The listing builds one solid part. Answer for the finished solid, in the listing's coordinates (mm). A direction names the side the tool comes from. Give positions to 0.01 mm unless a question says otherwise; leave off trailing zeros. Order: outer loops, then holes, each group sorted by start corner. A loop starts at its lowest first (then second) coordinate and runs counter-clockwise, first axis right, second up. Notation, with made-up numbers: (-36, 83.25) - (-29, 83.25) arc R17 ccw to (-29, 111.25) - close; hole circle Ø8 at (38.5, 79.25). An arc over 180 degrees is marked (long way). Write each question's results on one line, items separated by ' | '. Start each with the question number.
1. Section C-C (z = -12) is taken. Give the vertices of the cut face in (x, y), and give its area (3 significant figures).
2. Find the intervals of material crossed by L1, parallel to X at y = 43, z = 0; L2, parallel to X at y = 44.5, z = 44; L3, parallel to Z at x = -42, y = 34.5, in increasing order.
3. Flat-ended cylindrical pins translate along their axes: pin 1 (2 mm diameter, centred on x = -5.5, z = 67, fed in from +Y); pin 2 (1.5 mm diameter, centred on y = 32.5, z = 55, fed in from +X); pin 3 (3.5 mm diameter, centred on y = 47.5, z = 67.5, fed in from +X). Find the tip coordinate at first contact, or state that the pin passes through.
4. Section D-D (z = 61) is taken. Give the vertices of the cut face in (x, y).
5. Section A-A (y = 7.5) is taken. Give the vertices of the cut face in (x, z).
6. Which of the six approach directions +Z, -Z, +X, -X, +Y, -Y give full straight-line access (tool end or side, diameter ignored) to faces 4 (the face through (-1, 28, -65)), 5 (the face through (-15, 46, 69)), 6 (the face through (66.297, 2.535, -65.986))?
7. Section B-B (x = 34.5) is taken. Give the vertices of the cut face in (y, z), and give its area (3 significant figures).
8. Determine the mould class of faces 1 (the face through (-1, 0, -1)), 2 (the face through (-1, 25, 72)), 3 (the face through (52, 28, 1)) for opening direction Z: released by +Z, released by -Z, zero draft, split by the parting line, or undercut.
from build123d import *

# Parameters (mm, degrees)
SKETCH1_W           = 144
SKETCH1_H           = 144
BOSS_EXTRUDE1_DEPTH = 5
FILLET1_R           = 20
BOSS_EXTRUDE2_START = 45
SKETCH2_W           = 104
SKETCH2_H           = 130
BOSS_EXTRUDE2_DEPTH = 45
SKETCH3_R           = 1.5
CUT_EXTRUDE1_DEPTH  = 13
SKETCH5_W           = 15
SKETCH5_H           = 8
CUT_EXTRUDE2_DEPTH  = 8


with BuildPart() as part:
    # Sketch1 → Boss-Extrude1 (new body)
    with BuildSketch(Plane(origin=(0, 0, 0), x_dir=(1, 0, 0), z_dir=(0, 1, 0))):
        Rectangle(SKETCH1_W, SKETCH1_H)
    extrude(amount=BOSS_EXTRUDE1_DEPTH)

    # Fillet1
    fillet1_edges = [part.edges().sort_by_distance(p)[0] for p in [
        (72, 2.5, 72),
        (-72, 2.5, 72),
        (-72, 2.5, -72),
        (72, 2.5, -72),
    ]]
    fillet(fillet1_edges, radius=FILLET1_R)

    # Sketch2 → Boss-Extrude2 (add)
    with BuildSketch(Plane(origin=(0, 5, 0), x_dir=(1, 0, 0), z_dir=(0, 1, 0)).offset(BOSS_EXTRUDE2_START)):
        with BuildLine():
            Line((-72, 52), (-72, -52))
            ThreePointArc((-72, -52), (-66.142135624, -66.142135624), (-52, -72))
            Line((-52, -72), (52, -72))
            ThreePointArc((52, -72), (66.142135624, -66.142135624), (72, -52))
            Line((72, -52), (72, 62))
            ThreePointArc((72, 62), (69.071067812, 69.071067812), (62, 72))
            Line((62, 72), (-52, 72))
            ThreePointArc((-52, 72), (-66.142135624, 66.142135624), (-72, 52))
        make_face()
        Rectangle(SKETCH2_W, SKETCH2_H, mode=Mode.SUBTRACT)
    extrude(amount=-BOSS_EXTRUDE2_DEPTH)

    # Sketch3 → Cut-Extrude1 (cut)
    with BuildSketch(Plane(origin=(0, 50, 0), x_dir=(1, 0, 0), z_dir=(0, 1, 0))):
        with Locations(Location((-67, 0, 0), (0, 0, 270))):
            Circle(SKETCH3_R)
        with Locations(Location((67, 0, 0), (0, 0, 270))):
            Circle(SKETCH3_R)
    extrude(amount=-CUT_EXTRUDE1_DEPTH, mode=Mode.SUBTRACT)

    # Sketch5 → Cut-Extrude2 (cut)
    with BuildSketch(Plane.XY.offset(72)):
        with Locations((-7.5, 46)):
            Rectangle(SKETCH5_W, SKETCH5_H)
    extrude(amount=-CUT_EXTRUDE2_DEPTH, mode=Mode.SUBTRACT)


solid = part.part
Reported:
1) outline: (-72, 0) - (72, 0) - (72, 50) - (52, 50) - (52, 5) - (-52, 5) - (-52, 50) - (-72, 50) - close | area: 2,520 mm²
2) L1: -72 to -68.5, -65.5 to -52, 52 to 65.5, 68.5 to 72 | L2: -72 to -52, 52 to 72 | L3: -72 to -65, 65 to 72
3) pin 1: y = 42 | pin 2: x = 71.87 | pin 3: x = 66.52
4) outline: (-69.86, 0) - (69.86, 0) - (69.86, 50) - (52, 50) - (52, 5) - (-52, 5) - (-52, 50) - (-69.86, 50) - close
5) outline: (-72, -52) arc R20 ccw to (-52, -72) - (62, -72) arc R10 ccw to (72, -62) - (72, 52) arc R20 ccw to (52, 72) - (-52, 72) arc R20 ccw to (-72, 52) - close; hole (-52, -65) - (52, -65) - (52, 65) - (-52, 65) - close
6) face 4: +Y | face 5: +Z, +Y | face 6: -Z, +X, -Y
7) outline: (0, -72) - (50, -72) - (50, -65) - (5, -65) - (5, 65) - (50, 65) - (50, 72) - (0, 72) - close | area: 1,350 mm²
8) face 1: zero draft | face 2: released by +Z | face 3: undercut
